Autodesk Fusion 360 part; units mm, degrees
sketch "Sketch1" plane through (0, 0, 0) normal (0, 0, 1) x (1, 0, 0)
  line L0 (0, 0) -> (0, 11)
  line L1 (0, 11) -> (1.5, 11)
  line L2 (1.5, 11) -> (3, 9)
  line L3 (3, 9) -> (3, 0)
  line L4 (3, 0) -> (0, 0)
  dimension "d1" = 9
  dimension "d2" = 11
  dimension "d3" = 1.5
  dimension "d4" = 3
revolve "Revolve1" add sketch "Sketch1" angle 360 about axis through (0, 0, 0) along (0, 1, 0)
sketch "Sketch2" plane through (0, 0, 0) normal (0, 0, 1) x (1, 0, 0)
  line L0 (0.5, -1) -> (-0.5, -1)
  line L1 (-0.5, -1) -> (-0.5, 1)
  line L2 (-0.5, 1) -> (0.5, 1)
  line L3 (0.5, 1) -> (0.5, -1)
  line L4 (0.5, -1) -> (-0.5, 1) construction
  line L5 (-0.5, -1) -> (0.5, 1) construction
  dimension "d6" = 1
  dimension "d7" = 2
extrude "Extrude1" cut sketch "Sketch2" along normal through all and the other way through all
chamfer "Chamfer1" distance 0.5 angle 45 2 edges at (3, 0, 0) (-3, 0, 0)
thread "Thread1" thread offset 0 thread length 10
Input: part model. Units: mm. Frame: model coordinates. A direction names the side the tool comes from. Round coordinates to 2 decimals unless told otherwise and drop trailing zeros. Loops run counter-clockwise (first coordinate to the right, second up) from the corner with the lowest first, then second, coordinate; pieces in that order, holes last. Notation, with made-up numbers: (35.5, 24) - (71.5, 24) arc R13 cw to (71.5, 31) - close; hole circle Ø7 at (63.5, 36.5). An arc over 180 degrees is marked (long way). One line per item, written item: value. Start each with the question number.
(1) Ray query, line 1 (X direction, y = 6.25, z = -0.5); line 2 (Z direction, x = -1.15, y = 9.75); line 3 (X direction, y = 7, z = 1.05). Return the intervals inside material, ascending. Write a range as [from, to].
(2) Access query for faces 1 (the flat face through (0, 1, 0)), 2 (the cylindrical face through (2.86, 4.44, 0.9)). Directions: +Z, -Z, +X, -X, +Y, -Y. A direction counts if a zero-diameter tool reaches every point of the face in a straight line with its end or side. Return the directions, or none.
(3) Section B-B, the plane x = 0. Return loops of the section in (y, z), plus the area to 3 significant figures.
(4) Section C-C, the plane y = 2.5. Return loops of the section in (x, z), plus the area to 3 significant figures.
(5) Section D-D, the plane y = 9.5. Return loops of the section in (x, z) (3 decimals).
(6) Section A-A, the plane z = 0. Return loops of the section in (x, y).
(7) Contact query for flat-ended pins moving along their axis: P1, Ø2, axis at y = 9.5, z = 0.5, coming from the -X side; P2, Ø1.5, axis at y = 2.5, z = 2, coming from the +X side; P3, Ø1.5, axis at x = 2.5, z = 0.5, coming from the +Y side; P4, Ø1, axis at x = -2, y = 4.5, coming from the -Z side. Output: stop coordinate, or through.
(8) Draft query along X for faces 3 (the flat face through (0.5, 0.5, 0)), 4 (the flat face through (-0.5, 0.5, 0)), 5 (the conical face through (-0.35, 10.87, -1.56)), 6 (the flat face through (0, 11, 0)). Return one class per face: +X half, -X half, draft (parallel to the pull), parting line (faces both ways), or undercut.
Results below:
1. line 1: [-2.96, 2.96]
1. line 2: [-2.15, 2.15]
1. line 3: [-2.81, 2.81]
2. face 1: +Z, -Z, -Y
2. face 2: +Y, -Y
3. outline: (1, -3) - (9, -3) - (11, -1.5) - (11, 1.5) - (9, 3) - (1, 3) - close
3. area: 57.0 mm^2
4. outline: circle Ø6 at (0, 0)
4. area: 28.3 mm^2
5. outline: circle Ø5.25 at (0, 0)
6. outline: (-3, 0.5) - (-2.5, 0) - (-0.5, 0) - (-0.5, 1) - (0.5, 1) - (0.5, 0) - (3, 0) - (3, 9) - (1.5, 11) - (-1.5, 11) - (-3, 9) - close
7. P1: x = -3
7. P2: x = 2.73
7. P3: y = 10.6
7. P4: z = -2.6
8. face 3: undercut
8. face 4: undercut
8. face 5: parting line
8. face 6: draft
